Verification items for the finished model (mm, model axes). Face numbers are marked on the shaded views. Round coordinates to 2 decimals unless told otherwise and drop trailing zeros. Order: outer loops, then holes, each group sorted by start corner. A loop starts at its lowest first (then second) coordinate and runs counter-clockwise, first axis right, second up.
```python
from build123d import *

# Parameters (mm, degrees)
SKETCH1_W           = 12
SKETCH1_H           = 60
BOSS_EXTRUDE1_DEPTH = 4
SKETCH2_W           = 7.5
SKETCH2_H           = 21
CUT_EXTRUDE1_DEPTH  = 2
SKETCH4_R           = 3.5
BOSS_EXTRUDE2_DEPTH = 1
SKETCH5_R           = 16.5
BOSS_EXTRUDE3_DEPTH = 4
FILLET2_R           = 5


with BuildPart() as part:
    # Sketch1 → Boss-Extrude1 (new body)
    with BuildSketch(Plane(origin=(0, 0, 0), x_dir=(1, 0, 0), z_dir=(0, 1, 0))):
        Rectangle(SKETCH1_W, SKETCH1_H)
    extrude(amount=BOSS_EXTRUDE1_DEPTH)

    # Sketch2 → Cut-Extrude1 (cut)
    with BuildSketch(Plane(origin=(0, 4, 0), x_dir=(1, 0, 0), z_dir=(0, 1, 0))):
        with Locations((0, -14.685)):
            Rectangle(SKETCH2_W, SKETCH2_H)
    extrude(amount=-CUT_EXTRUDE1_DEPTH, mode=Mode.SUBTRACT)

    # Sketch4 → Boss-Extrude2 (add)
    with BuildSketch(Plane.XZ):
        with Locations((0, 21.18)):
            Circle(SKETCH4_R)
    extrude(amount=BOSS_EXTRUDE2_DEPTH)

    # Sketch5 → Boss-Extrude3 (add)
    with BuildSketch(Plane(origin=(0, 4, 0), x_dir=(1, 0, 0), z_dir=(0, 1, 0))):
        with Locations((0, 21.19)):
            Circle(SKETCH5_R)
    extrude(amount=-BOSS_EXTRUDE3_DEPTH)

    # Fillet2
    fillet2_edges = [part.edges().sort_by_distance(p)[0] for p in [
        (6, 2, 30),
        (-6, 2, 30),
    ]]
    fillet(fillet2_edges, radius=FILLET2_R)


solid = part.part
```
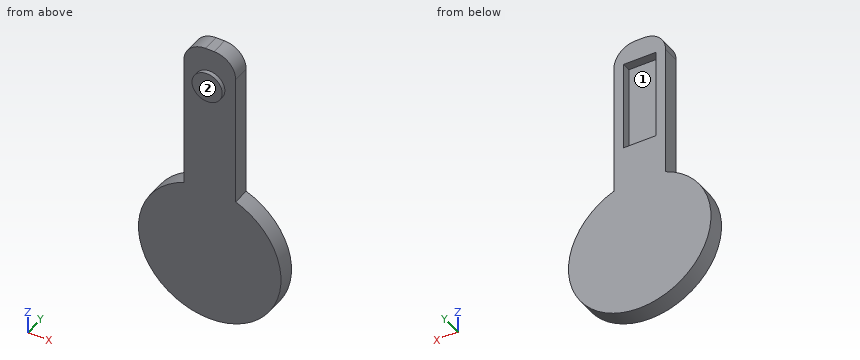
1) Sectioned sample at C-C on x = 0. Record the cut outline in (y, z) (3 decimals).
2) Sectioned sample at D-D on z = -21.19. Record the cut outline in (x, y), then the cut area to 3 significant figures.
3) Go/stop test with flat-tipped pins: pin 1 Ø10 at (x, z) = (-0.5, 5) entering from -Y; pin 2 Ø2 at (y, z) = (1, -1.5) entering from +X; pin 3 Ø1.5 at (x, y) = (-4, 1) entering from +Z; pin 4 Ø1.5 at (x, z) = (8, 17) entering from -Y. Record where each tip stops, or that it passes through.
4) Sectioned sample at A-A on y = 2.7. Record the cut outline in (x, z) (3 decimals).
5) Sectioned sample at B-B on z = 15. Record the cut outline in (x, y), then the cut area to 3 significant figures.
6) Draft check along X on the marked faces 1 and 2. Enter one of: released by +X, released by -X, zero draft, split by the parting line, or undercut.
7) Scan lines: probe 1 along X at (y, z) = (2.25, 12); probe 2 along X at (y, z) = (0.2, 23); probe 3 along Y at (x, z) = (-4.5, -21.5). Record each from-to range of solid material in increasing order.
Returned:
1. outline: (-1, 17.68) - (0, 17.68) - (0, -37.69) - (4, -37.69) - (4, 4.185) - (2, 4.185) - (2, 25.185) - (4, 25.185) - (4, 30) - (0, 30) - (0, 24.68) - (-1, 24.68) - close
2. outline: (-16.5, 0) - (16.5, 0) - (16.5, 4) - (-16.5, 4) - close
2. area: 132 mm2
3. pin 1: stops at y = 0
3. pin 2: stops at x = 6
3. pin 3: stops at z = 29.47
3. pin 4: passes through
4. outline: (-6, -5.82) arc R16.5 ccw (long way) to (6, -5.82) - (6, 25) arc R5 ccw to (1, 30) - (-1, 30) arc R5 ccw to (-6, 25) - close; hole (-3.75, 4.185) - (3.75, 4.185) - (3.75, 25.185) - (-3.75, 25.185) - close
5. outline: (-6, 0) - (6, 0) - (6, 4) - (3.75, 4) - (3.75, 2) - (-3.75, 2) - (-3.75, 4) - (-6, 4) - close
5. area: 33.0 mm2
6. face 1: undercut
6. face 2: zero draft
7. probe 1: x = -6 to -3.75, 3.75 to 6
7. probe 2: x = -6 to 6
7. probe 3: y = 0 to 4
